Read the model definition and answer for the solid it produces. Units are mm, in the model's axes. Face numbers are marked on the shaded views. Coordinates: 2 decimals unless noted, no trailing zeros. Write each loop counter-clockwise with the first axis right and the second up, starting at its lowest first coordinate (ties: lowest second). Pieces come first, ordered by that corner, then holes.
Item 1: Determine the mould class of the marked faces 1, 2 and 3 for opening direction X: released by +X, released by -X, zero draft, split by the parting line, or undercut.
Item 2: This flat-tipped pin is pushed along its axis until it touches: P1, Ø5, axis at y = -428.5, z = 41.5, coming from the +X side. Where does it stop, or does it pass through?
Item 3: Section B-B (z = -22.5) is taken. Give the vertices of the cut face in (x, y).
Item 4: Section C-C (y = -233) is taken. Give the vertices of the cut face in (x, z).
Item 5: Section A-A (x = -34.5) is taken. Give the vertices of the cut face in (y, z), then the cut area to 3 significant figures.
Item 6: Straight lines are drawn through the part: probe 1 along X at (y, z) = (-302, -24.5); probe 2 along Y at (x, z) = (-34, 29); probe 3 along X at (y, z) = (-417, 29). For each, find the intervals that lie inside material, in ascending order.
from build123d import *

# Parameters (mm, degrees)
F0_W     = 102.922255
F0_H     = 77.739151
F1_DEPTH = 508
F2_R     = 25.4
F4_D     = 55.88
F5_SIZE  = 12.7


with BuildPart() as f1:
    # F0 (on Front) → F1 (new body)
    with BuildSketch(Plane.XZ):
        with Locations((-26.825475, 10.584204)):
            Rectangle(F0_W, F0_H)
    extrude(amount=F1_DEPTH)

    # F2
    f2_edges = [f1.edges().sort_by_distance(p)[0] for p in [
        (24.635652, -254, 49.45378),
    ]]
    fillet(f2_edges, radius=F2_R)

    # F4 (through all)
    with Locations(Plane.XY.offset(49.45378)):
        with Locations((-26.449531, -303.084731)):
            Hole(F4_D / 2)

    # F5
    f5_edges = [f1.edges().sort_by_distance(p)[0] for p in [
        (-39.525476, -508, 49.45378),
        (17.196164, -508, 42.014292),
        (-78.286603, -508, 10.584204),
        (24.635652, -508, -2.115796),
        (-26.825476, -508, -28.285371),
    ]]
    chamfer(f5_edges, length=F5_SIZE)


solid = f1.part
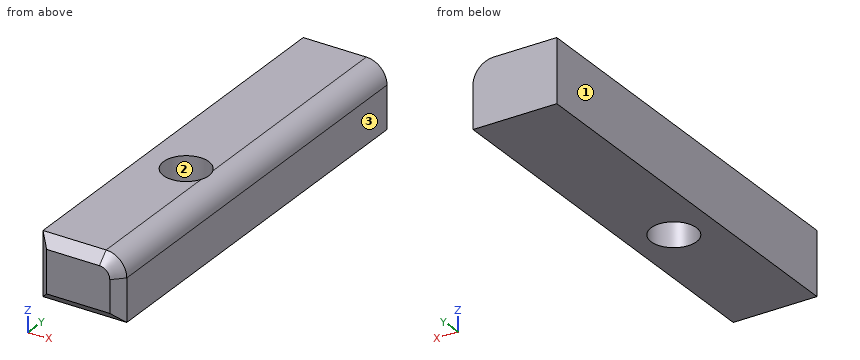
Established:
1. face 1: released by -X
1. face 2: undercut
1. face 3: released by +X
2. P1: stops at x = 19.77
3. outline: (-78.29, -495.3) - (-72.5, -501.09) - (18.85, -501.09) - (24.64, -495.3) - (24.64, 0) - (-78.29, 0) - close; hole circle Ø55.88 at (-26.45, -303.08)
4. outline: (-78.29, -28.29) - (24.64, -28.29) - (24.64, 24.05) arc R25.4 ccw to (-0.76, 49.45) - (-78.29, 49.45) - close
5. outline: (-508, -15.59) - (-495.3, -28.29) - (-329.84, -28.29) - (-329.84, 49.45) - (-495.3, 49.45) - (-508, 36.75) - close; (-276.33, -28.29) - (0, -28.29) - (0, 49.45) - (-276.33, 49.45) - close
5. area: 35,200 mm2
6. probe 1: x = -78.29 to -54.37, 1.47 to 24.64
6. probe 2: y = -508 to -329.99, -276.18 to 0
6. probe 3: x = -78.29 to 24.15
